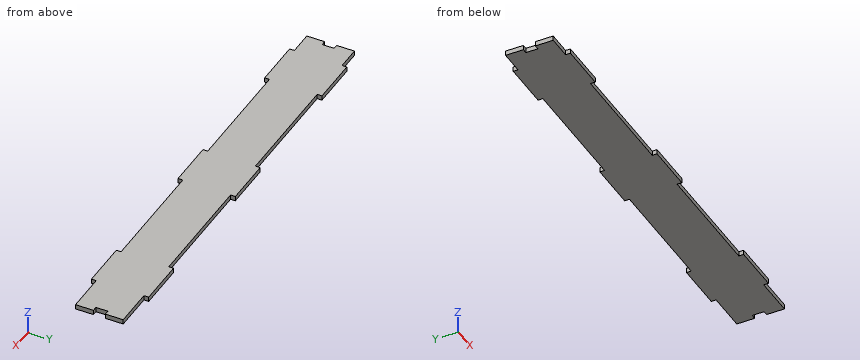
Autodesk Inventor part; units mm, degrees
ref_plane "Work Plane1" through (-283, -128.2, 0) normal (-1, 0, 0) x (0, 0, 1)
ref_plane "YZ Plane" through (0, 0, 0) normal (1, 0, 0) x (0, 1, 0)
ref_plane "XZ Plane" through (0, 0, 0) normal (0, 1, 0) x (-1, 0, 0)
sketch "Sketch2" plane through (0, 0, 0) normal (0, 0, 1) x (1, 0, 0)
  line L0 (-469, -128.2) -> (-449, -128.2)
  line L1 (-449, -128.2) -> (-449, -124.2)
  line L2 (-449, -124.2) -> (-409, -124.2)
  line L3 (-409, -124.2) -> (-409, -128.2)
  line L4 (-409, -128.2) -> (-309.6667, -128.2)
  line L5 (-309.6667, -128.2) -> (-309.6667, -124.2)
  line L6 (-309.6667, -124.2) -> (-269.6667, -124.2)
  line L7 (-269.6667, -124.2) -> (-269.6667, -128.2)
  line L8 (-269.6667, -128.2) -> (-170.3333, -128.2)
  line L9 (-170.3333, -128.2) -> (-170.3333, -124.2)
  line L10 (-170.3333, -124.2) -> (-130.3333, -124.2)
  line L11 (-130.3333, -124.2) -> (-130.3333, -128.2)
  line L12 (-130.3333, -128.2) -> (-101, -128.2)
  line L13 (-101, -128.2) -> (-97, -128.2)
  line L14 (-97, -128.2) -> (-97, -168.2)
  line L15 (-469, -128.2) -> (-469, -168.2)
  line L16 (-469, -148.2) -> (-513.1523, -148.2)
  line L17 (-170.3333, -168.2) -> (-170.3333, -172.2)
  line L18 (-309.6667, -168.2) -> (-309.6667, -172.2)
  line L19 (-130.3333, -172.2) -> (-130.3333, -168.2)
  line L20 (-449, -172.2) -> (-409, -172.2)
  line L21 (-449, -168.2) -> (-449, -172.2)
  line L22 (-409, -172.2) -> (-409, -168.2)
  line L23 (-269.6667, -172.2) -> (-269.6667, -168.2)
  line L24 (-309.6667, -172.2) -> (-269.6667, -172.2)
  line L25 (-170.3333, -172.2) -> (-130.3333, -172.2)
  line L26 (-449, -168.2) -> (-469, -168.2)
  line L27 (-309.6667, -168.2) -> (-409, -168.2)
  line L28 (-97, -168.2) -> (-130.3333, -168.2)
  line L29 (-170.3333, -168.2) -> (-269.6667, -168.2)
  point P0 (0, 0)
  dimension "d2" = 4
  dimension "d3" = 40
extrude "Extrusion2" add sketch "Sketch2" along normal blind 4
sketch "Sketch4" plane through (0, 0, 4) normal (0, 0, 1) x (1, 0, 0)
  line L0 (-170.3333, -128.2) -> (-269.6667, -128.2)
  line L1 (-269.6667, -128.2) -> (-269.6667, -124.2)
  line L2 (-269.6667, -124.2) -> (-309.6667, -124.2)
  line L3 (-309.6667, -124.2) -> (-309.6667, -128.2)
  line L4 (-309.6667, -128.2) -> (-409, -128.2)
  line L5 (-409, -128.2) -> (-409, -124.2)
  line L6 (-409, -124.2) -> (-449, -124.2)
  line L7 (-449, -124.2) -> (-449, -128.2)
  line L8 (-449, -128.2) -> (-469, -128.2)
  line L9 (-469, -128.2) -> (-469, -168.2)
  line L10 (-469, -168.2) -> (-449, -168.2)
  line L11 (-449, -168.2) -> (-449, -172.2)
  line L12 (-449, -172.2) -> (-409, -172.2)
  line L13 (-409, -172.2) -> (-409, -168.2)
  line L14 (-409, -168.2) -> (-309.6667, -168.2)
  line L15 (-309.6667, -168.2) -> (-309.6667, -172.2)
  line L16 (-309.6667, -172.2) -> (-269.6667, -172.2)
  line L17 (-269.6667, -172.2) -> (-269.6667, -168.2)
  line L18 (-269.6667, -168.2) -> (-170.3333, -168.2)
  line L19 (-170.3333, -168.2) -> (-170.3333, -172.2)
  line L20 (-170.3333, -172.2) -> (-130.3333, -172.2)
  line L21 (-130.3333, -172.2) -> (-130.3333, -168.2)
  line L22 (-130.3333, -168.2) -> (-97, -168.2)
  line L23 (-97, -168.2) -> (-97, -128.2)
  line L24 (-97, -128.2) -> (-130.3333, -128.2)
  line L25 (-130.3333, -128.2) -> (-130.3333, -124.2)
  line L26 (-130.3333, -124.2) -> (-170.3333, -124.2)
  line L27 (-170.3333, -124.2) -> (-170.3333, -128.2)
  line L28 (-469, -143.2) -> (-465, -143.2)
  line L29 (-465, -143.2) -> (-465, -153.2)
  line L30 (-465, -153.2) -> (-469, -153.2)
  line L31 (-469, -153.2) -> (-469, -143.2)
  line L32 (-469, -128.2) -> (-469, -168.2)
  point P0 (0, 0)
  point P1 (-469, -148.2)
  dimension "d13" = 4
  dimension "d14" = 10
  dimension "d17" = 40
  dimension "d18" = 15
extrude "Extrusion4" cut sketch "Sketch4" against normal blind 4 contours L28 L29 L30 L9
ref_plane "Work Plane1" through (-283, -128.2, 0) normal (-1, 0, 0) x (0, 0, 1)
mirror "Mirror1" about plane through (-283, -128.2, 0) normal (-1, 0, 0) of "Extrusion4"
properties part number "F6"
Here's how the part is built. I have some questions about the finished solid (model axes, mm). Coordinates: 2 decimals unless noted, no trailing zeros. Order: outer loops, then holes, each group sorted by start corner. A loop starts at its lowest first (then second) coordinate and runs counter-clockwise, first axis right, second up. Notation, with made-up numbers: M -11,31 L -6,31 A20 ccw -6,38 Z; hole C 65.5,33 d7. An arc over 180 degrees is marked long. Answer as CSV lines item,"result". Start each with the question number.
1. I need wall thicknesses on line 1 (X direction, y = -127, z = 1.7); line 2 (Y direction, x = -172, z = 1.7); line 3 (X direction, y = -153, z = 1.1). Which ranges of each line are inside material? Lowest first, please. Write a range as [from, to].
2. I want a section at A-A, the plane x = -356.5. Write out the boundary of the cut face in (y, z), and give its area (3 significant figures).
3. For pin 1 (2 mm diameter, centred on x = -383, z = 3, fed in from +Y); pin 2 (2 mm diameter, centred on y = -170.5, z = 1, fed in from +X); pin 3 (2 mm diameter, centred on y = -150, z = 2.5, fed in from -X); pin 4 (6 mm diameter, centred on x = -205.5, y = -162.5, fed in from -Z), each with a flat end and sliding along its axis, tell me the tip position at first contact or that it passes through.
4. I want a section at B-B, the plane y = -150. Write out the boundary of the cut face in (x, z).
Recorded:
1,line 1,"x = [-449, -409], [-309.67, -269.67], [-170.33, -130.33]"
1,line 2,"y = [-168.2, -128.2]"
1,line 3,"x = [-465, -101]"
2,outline,"M -168.2,0 L -128.2,0 L -128.2,4 L -168.2,4 Z"
2,area,"160 mm2"
3,pin 1,"stops at y = -128.2"
3,pin 2,"stops at x = -130.33"
3,pin 3,"stops at x = -465"
3,pin 4,"stops at z = 0"
4,outline,"M -465,0 L -101,0 L -101,4 L -465,4 Z"
